Study the drawing (mm; zero at the part's minimum x, y, z) and answer. Round coordinates to 2 decimals unless told otherwise and drop trailing zeros. Loops run counter-clockwise (first coordinate to the right, second up) from the corner with the lowest first, then second, coordinate; pieces in that order, holes last. Notation, with made-up numbers: (45, 0.5) -> (61, 0.5) arc R15 cw to (61, 14.5) -> close; hole circle Ø6 at (78.5, 4). An arc over 180 degrees is marked (long way). Write each question's results on one line, items separated by ' | '. Start each with the question number.
(1) Flat-ended cylindrical pins translate along their axes: pin 1 (1.5 mm diameter, centred on x = 123.5, y = 3.5, fed in from -Z); pin 2 (12 mm diameter, centred on x = 45, z = 69.5, fed in from +Y); pin 3 (2.5 mm diameter, centred on x = 62, y = 3.5, fed in from +Z); pin 4 (4 mm diameter, centred on x = 125, z = 75, fed in from -Y). Find the tip coordinate at first contact, or state that the pin passes through.
(2) The part is cut by section C-C (z = 82). Determine the outline of the cut face in (x, y), plus the area to 3 significant figures.
(3) Straight lines are drawn through the part: probe 1 along X at (y, z) = (2.35, 20); probe 2 along Z at (x, y) = (240, 1.25); probe 3 along X at (y, z) = (0.7, 9). For each, find the intervals that lie inside material, in ascending order.
(4) The part is cut by section D-D (y = 3.8). Count the separate pieces of the cut face and the enclosed holes in it, plus the area to 3 significant figures.
(5) The part is cut by section A-A (x = 167). Determine the outline of the cut face in (y, z).
(6) The part is cut by section B-B (z = 125). Determine the outline of the cut face in (x, y).
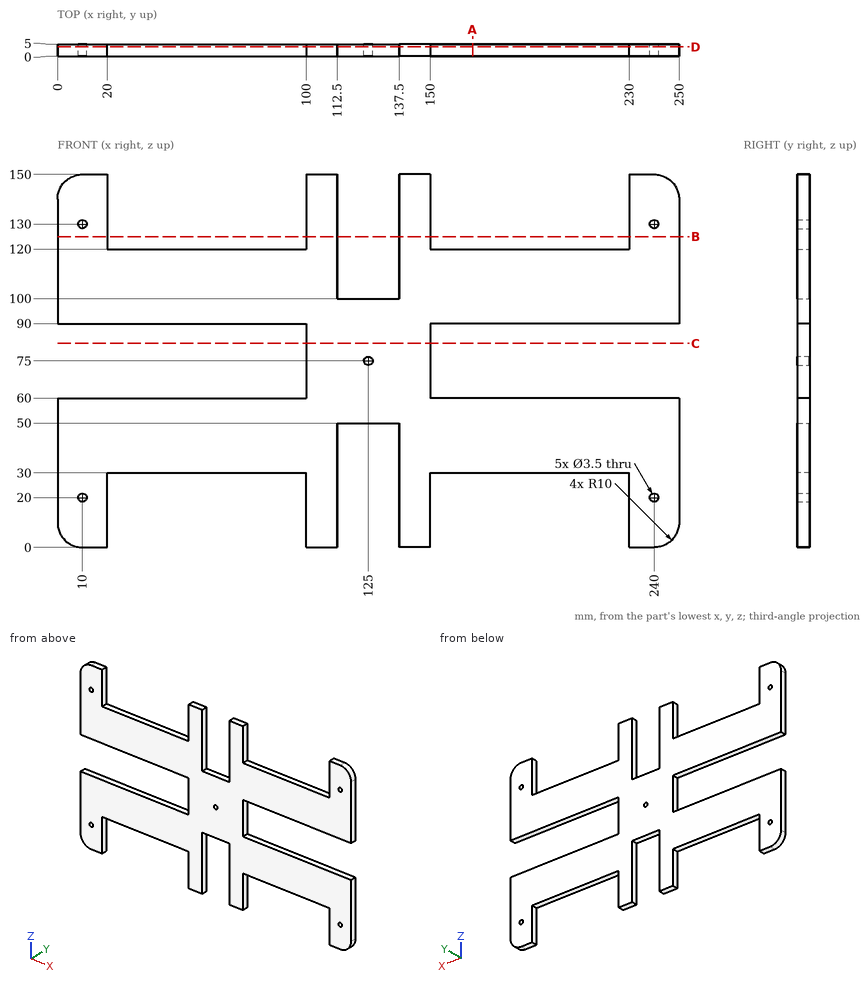
Checked values:
1) pin 1: stops at z = 50 | pin 2: passes through | pin 3: stops at z = 120 | pin 4: stops at y = 0
2) outline: (100, 0) -> (150, 0) -> (150, 5) -> (100, 5) -> close | area: 250 mm2
3) probe 1: x = 0 to 8.25, 11.75 to 20, 100 to 112.5, 137.5 to 150, 230 to 238.25, 241.75 to 250 | probe 2: z = 0 to 18.25, 21.75 to 60, 90 to 128.25, 131.75 to 150 | probe 3: x = 0.05 to 20, 100 to 112.5, 137.5 to 150, 230 to 249.95
4) separate pieces: 1 | enclosed holes: 5 | area: 19,300 mm2
5) outline: (0, 30) -> (5, 30) -> (5, 60) -> (0, 60) -> close; (0, 90) -> (5, 90) -> (5, 120) -> (0, 120) -> close
6) outline: (0, 0) -> (20, 0) -> (20, 5) -> (0, 5) -> close; (100, 0) -> (112.5, 0) -> (112.5, 5) -> (100, 5) -> close; (137.5, 0) -> (150, 0) -> (150, 5) -> (137.5, 5) -> close; (230, 0) -> (250, 0) -> (250, 5) -> (230, 5) -> close
